Geometry check sheet. Reference: the model listing, model coordinates, mm. A direction names the side the tool comes from. Coordinates: 2 decimals unless noted, no trailing zeros. Write each loop counter-clockwise with the first axis right and the second up, starting at its lowest first coordinate (ties: lowest second). Pieces come first, ordered by that corner, then holes.
Autodesk Inventor part; units mm, degrees
sketch "Sketch1" plane through (0, 0, 0) normal (0, 1, 0) x (-1, 0, 0)
  line L0 (10, -10) -> (-10, -10)
  line L1 (-10, -10) -> (-10, 10)
  line L2 (-10, 10) -> (10, 10)
  line L3 (10, 10) -> (10, -10)
  line L4 (0, -13.825) -> (0, 13.825)
  line L5 (-14, 0) -> (14, 0)
  point P0 (0, 0)
  point P1 (0, -10)
  point P2 (10, 0)
  dimension "d0" = 20
  dimension "d1" = 20
extrude "Extrusion1" add sketch "Sketch1" along normal mid plane 1
sketch "Sketch2" plane through (0, -0.5, 0) normal (0, -1, 0) x (1, 0, 0)
  circle A0 centre (-5, 5) radius 2.5
  line L0 (10, 10) -> (-10, 10)
  line L1 (-10, 10) -> (-10, -10)
  circle A1 centre (5, -5) radius 2.5
  point P0 (0, 0)
  dimension "d4" = 5
  dimension "d5" = 5
  dimension "d6" = 5
  dimension "d9" = 360
extrude "Extrusion2" add sketch "Sketch2" along normal blind 2.5
sketch "Sketch3" plane through (0, 0.5, 0) normal (0, 1, 0) x (1, 0, 0)
  circle A0 centre (0, 0) radius 5
  dimension "d13" = 10
extrude "Extrusion3" add sketch "Sketch3" along normal blind 25
sketch "Sketch7" plane through (0, 25.5, 0) normal (0, 1, 0) x (1, 0, 0)
  circle A0 centre (0, 0) radius 2.5
  dimension "d50" = 5
extrude "Extrusion4" add sketch "Sketch7" along normal blind 5
properties part number "Tree_Trunk"
1. Access from +Z, -Z, +X, -X, +Y, -Y to the whole of each face (thin tool, end or side, straight path). Record for faces 1 (the flat face through (10, 0, 0)), 2 (the flat face through (2, 0.5, 5)), 3 (the cylindrical face through (-2.615, -1.732, 4.249)).
Computed values:
face 1: +Z, -Z, +X, +Y, -Y
face 2: +Y
face 3: -Y
2. Thickness scan on line 1 along Y through (x, z) = (-2.75, -9); line 2 along Y through (x, z) = (-3.5, -3.5); line 3 along X through (y, z) = (2.5, 2.25). Record the ranges inside material, lowest first.
Computed values:
line 1: y = -0.5 to 0.5
line 2: y = -0.5 to 25.5
line 3: x = -4.47 to 4.47
3. Sectioned sample at A-A, the plane x = -3. Record the boundary of the cut face in (y, z), and give its area (4 significant figures).
Computed values:
outline: (-3, 3.5) - (-0.5, 3.5) - (-0.5, -10) - (0.5, -10) - (0.5, -4) - (25.5, -4) - (25.5, 4) - (0.5, 4) - (0.5, 10) - (-0.5, 10) - (-0.5, 6.5) - (-3, 6.5) - close
area: 227.5 mm2
4. Gauge pin test, flat ends, axial feed: pin 1 Ø4 at (x, y) = (7.5, 5.5) entering from +Z; pin 2 Ø3 at (x, y) = (-4, 24.5) entering from -Z; pin 3 Ø3 at (x, z) = (-5.5, 5.5) entering from +Y; pin 4 Ø6 at (y, z) = (19, 4) entering from -X. Record the tip position at first contact, or that the pin passes through.
Computed values:
pin 1: passes through
pin 2: stops at z = -4.33
pin 3: stops at y = 0.5
pin 4: stops at x = -4.9
5. Sectioned sample at B-B, the plane z = 0. Record the boundary of the cut face in (x, y).
Computed values:
outline: (-10, -0.5) - (10, -0.5) - (10, 0.5) - (5, 0.5) - (5, 25.5) - (2.5, 25.5) - (2.5, 30.5) - (-2.5, 30.5) - (-2.5, 25.5) - (-5, 25.5) - (-5, 0.5) - (-10, 0.5) - close
6. Sectioned sample at D-D, the plane x = -6.75. Record the boundary of the cut face in (y, z), and give its area (3 significant figures).
Computed values:
outline: (-3, 3.21) - (-0.5, 3.21) - (-0.5, -10) - (0.5, -10) - (0.5, 10) - (-0.5, 10) - (-0.5, 6.79) - (-3, 6.79) - close
area: 28.9 mm2
7. Sectioned sample at C-C, the plane y = 28. Record the boundary of the cut face in (x, z).
Computed values:
outline: circle Ø5 at (0, 0)
